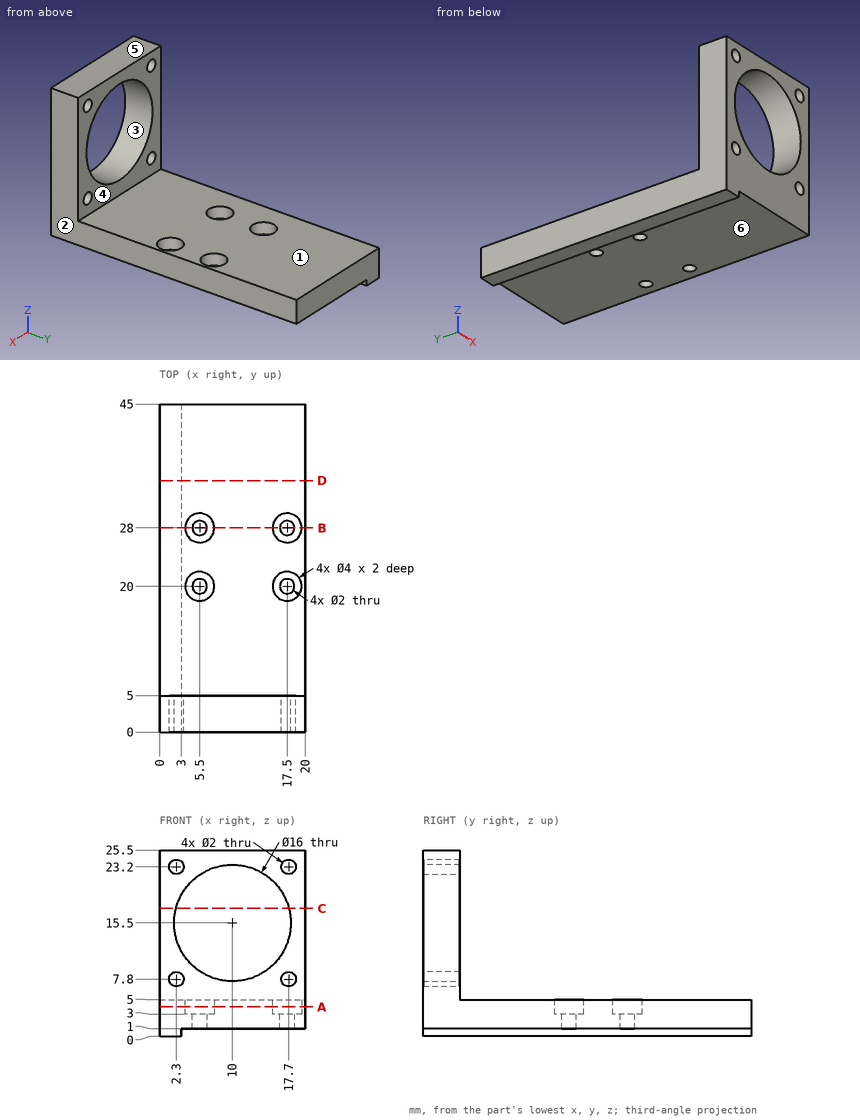
Answer from the drawing. Dimensions are ordinates in mm from the lowest x, y and z of the part. A direction names the side the tool comes from. Give positions to 0.01 mm unless a question says otherwise; leave off trailing zeros. Loops run counter-clockwise (first coordinate to the right, second up) from the corner with the lowest first, then second, coordinate; pieces in that order, holes last.
Item 1: A tool of negligible diameter and unlimited length cuts with its end or side. For the marked faces 4, 5 and 6, from which of +Z, -Z, +X, -X, +Y, -Y can it reach the whole face along a straight path? Write none if from no direction.
Derived:
face 4: +Z, +X, -X, +Y
face 5: +Z, +X, -X, +Y, -Y
face 6: -Z, +X, +Y, -Y
Item 2: Determine the mould class of the marked faces 1, 2 and 3 for opening direction X: +X half, -X half, draft (parallel to the pull), parting line (faces both ways), or undercut.
Derived:
face 1: draft
face 2: +X half
face 3: undercut
Item 3: Each of these flat-tipped pins is pushed along its axis until it touches: pin 1 Ø3 at (x, z) = (17.7, 23.2) entering from +Y; pin 2 Ø3 at (x, y) = (5.5, 28) entering from -Z; pin 3 Ø10 at (x, y) = (15.5, 12) entering from +Z. Where does it stop, or does it pass through?
Derived:
pin 1: stops at y = 5
pin 2: stops at z = 1
pin 3: stops at z = 5
Item 4: A cutting plane is placed at D-D (y = 34.5). Give the vertices of the cut face in (x, z), then the cut area to 3 significant figures.
Derived:
outline: (0, 0) - (3, 0) - (3, 1) - (20, 1) - (20, 5) - (0, 5) - close
area: 83.0 mm2
Item 5: A cutting plane is placed at B-B (y = 28). Give the vertices of the cut face in (x, z), then the cut area to 3 significant figures.
Derived:
outline: (0, 0) - (3, 0) - (3, 1) - (4.5, 1) - (4.5, 3) - (3.5, 3) - (3.5, 5) - (0, 5) - close; (6.5, 1) - (16.5, 1) - (16.5, 3) - (15.5, 3) - (15.5, 5) - (7.5, 5) - (7.5, 3) - (6.5, 3) - close; (18.5, 1) - (20, 1) - (20, 5) - (19.5, 5) - (19.5, 3) - (18.5, 3) - close
area: 59.0 mm2
Item 6: A cutting plane is placed at A-A (z = 4). Give the vertices of the cut face in (x, y).
Derived:
outline: (0, 0) - (20, 0) - (20, 45) - (0, 45) - close; hole circle Ø4 at (5.5, 20); hole circle Ø4 at (5.5, 28); hole circle Ø4 at (17.5, 20); hole circle Ø4 at (17.5, 28)
Item 7: A cutting plane is placed at C-C (z = 17.5). Give the vertices of the cut face in (x, y).
Derived:
outline: (0, 0) - (2.25, 0) - (2.25, 5) - (0, 5) - close; (17.75, 0) - (20, 0) - (20, 5) - (17.75, 5) - close
Item 8: Find the intervals of material crossed by line 1 along Y through (x, z) = (5.5, 1.65); line 2 along Y through (x, z) = (17.5, 4); line 3 along Y through (x, z) = (4.25, 23.25), in increasing order.
Derived:
line 1: y = 0 to 19, 21 to 27, 29 to 45
line 2: y = 0 to 18, 22 to 26, 30 to 45
line 3: y = 0 to 5
